Read the model definition and answer for the solid it produces. Units are mm, in the model's axes. Face numbers are marked on the shaded views. A direction names the side the tool comes from. Give positions to 0.01 mm unless a question says otherwise; leave off trailing zeros. Write each loop counter-clockwise with the first axis right and the second up, starting at its lowest first coordinate (ties: lowest second). Pieces come first, ordered by that corner, then holes.
```python
from build123d import *

# Parameters (mm, degrees)
SKETCH2_R           = 60.625
SKETCH2_R_2         = 45
BOSS_EXTRUDE1_DEPTH = 4.5
SKETCH3_R           = 49
SKETCH3_R_2         = 45
BOSS_EXTRUDE2_DEPTH = 52
SKETCH4_W           = 13.25
SKETCH4_H           = 8
SKETCH4_W_2         = 8
SKETCH4_H_2         = 38.5
BOSS_EXTRUDE3_DEPTH = 13
SKETCH5_W           = 10
SKETCH5_H           = 20
CUT_EXTRUDE1_DEPTH  = 26
SKETCH6_R           = 5
CUT_EXTRUDE2_DEPTH  = 50.375
SKETCH7_R           = 1.3
CUT_EXTRUDE3_DEPTH  = 7.2
BOSS_EXTRUDE4_DEPTH = 4
FILLET1_R           = 1
SKETCH9_R           = 2.5
CUT_EXTRUDE4_DEPTH  = 5.5000001


with BuildPart() as part:
    # Sketch2 → Boss-Extrude1 (new body)
    with BuildSketch(Plane(origin=(0, 0, 0), x_dir=(1, 0, 0), z_dir=(0, 1, 0))):
        Circle(SKETCH2_R)
        Circle(SKETCH2_R_2, mode=Mode.SUBTRACT)
    extrude(amount=BOSS_EXTRUDE1_DEPTH)

    # Sketch3 → Boss-Extrude2 (add)
    with BuildSketch(Plane(origin=(0, 4.5, 0), x_dir=(1, 0, 0), z_dir=(0, 1, 0))):
        Circle(SKETCH3_R)
        Circle(SKETCH3_R_2, mode=Mode.SUBTRACT)
    extrude(amount=BOSS_EXTRUDE2_DEPTH)

    # Sketch4 → Boss-Extrude3 (add, symmetric)
    with BuildSketch(Plane(origin=(0, 0, 0), x_dir=(0, 0, -1), z_dir=(1, 0, 0))):
        Polygon((-31.75, 30.5), (-45, 30.5), (-45, 17.25), align=None)
        with Locations((-38.375, 34.5)):
            Rectangle(SKETCH4_W, SKETCH4_H)
        with Locations((15.25, 19.25)):
            Rectangle(SKETCH4_W_2, SKETCH4_H_2)
    extrude(amount=BOSS_EXTRUDE3_DEPTH, both=True)

    # Sketch5 → Cut-Extrude1 (cut)
    with BuildSketch(Plane.XY):
        with Locations((0, 19.5)):
            Rectangle(SKETCH5_W, SKETCH5_H)
    extrude(amount=-CUT_EXTRUDE1_DEPTH, mode=Mode.SUBTRACT)

    # Sketch6 → Cut-Extrude2 (cut, through all)
    with BuildSketch(Plane.XY.offset(-11.25)):
        with Locations((0, 14)):
            Circle(SKETCH6_R)
    extrude(amount=-CUT_EXTRUDE2_DEPTH, mode=Mode.SUBTRACT)

    # Sketch7 → Cut-Extrude3 (cut)
    with BuildSketch(Plane(origin=(0, 38.5, 0), x_dir=(1, 0, 0), z_dir=(0, 1, 0))):
        with Locations((-5, 13.75)):
            Circle(SKETCH7_R)
        with Locations((5, 13.75)):
            Circle(SKETCH7_R)
        with Locations((-5, -34.25)):
            Circle(SKETCH7_R)
        with Locations((5, -34.25)):
            Circle(SKETCH7_R)
    extrude(amount=-CUT_EXTRUDE3_DEPTH, mode=Mode.SUBTRACT)

    # Sketch8 → Boss-Extrude4 (add)
    with BuildSketch(Plane.XZ):
        with BuildLine():
            Line((13, -11.25), (-13, -11.25))
            Line((-13, -11.25), (-37.248431585, -25.249838503))
            ThreePointArc((-37.248431585, -25.249838503), (0, -45), (37.248431585, -25.249838503))
            Line((37.248431585, -25.249838503), (13, -11.25))
        make_face()
        with BuildLine():
            Line((-19.516660498, -24.25), (-24.906460381, -27.361802413))
            ThreePointArc((-24.906460381, -27.361802413), (0, -37), (24.906460381, -27.361802413))
            Line((24.906460381, -27.361802413), (19.516660498, -24.25))
            Line((19.516660498, -24.25), (-19.516660498, -24.25))
        make_face(mode=Mode.SUBTRACT)
    extrude(amount=-BOSS_EXTRUDE4_DEPTH)

    # Fillet1
    fillet1_edges = [part.edges().sort_by_distance(p)[0] for p in [
        (-49, 4.5, 0),
    ]]
    fillet(fillet1_edges, radius=FILLET1_R)

    # Sketch9 → Cut-Extrude4 (cut, through all)
    with BuildSketch(Plane(origin=(0, 4.5, 0), x_dir=(1, 0, 0), z_dir=(0, 1, 0))):
        with Locations((35, 42)):
            Circle(SKETCH9_R)
        with Locations((35, -42)):
            Circle(SKETCH9_R)
        with Locations((-35, -42)):
            Circle(SKETCH9_R)
        with Locations((-35, 42)):
            Circle(SKETCH9_R)
    extrude(amount=-CUT_EXTRUDE4_DEPTH, mode=Mode.SUBTRACT)


solid = part.part
```
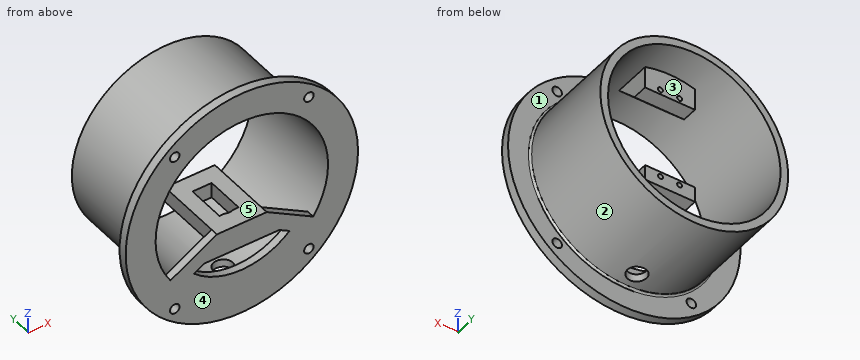
Item 1: Section D-D (y = 14) is taken. Write down the section's boundary in (x, z), and give its area (3 significant figures).
Result set:
outline: (-13, -19.25) - (-5, -19.25) - (-5, -11.25) - (-13, -11.25) - close; (-5, -48.74) - (-5, -44.72) arc R45 cw (long way) to (5, -44.72) - (5, -48.74) arc R49 ccw (long way) to start; (5, -19.25) - (13, -19.25) - (13, -11.25) - (5, -11.25) - close
area: 1,270 mm2
Item 2: Determine the mould class of the marked faces 1, 2 and 3 for opening direction X: pulls with the +X half, pulls with the -X half, needs draft (parallel to the pull), parting line crosses it, or undercut.
Result set:
face 1: needs draft
face 2: parting line crosses it
face 3: undercut
Item 3: Find the intervals of material crossed by line 1 along X through (y, z) = (30, 0); line 2 along Z through (x, y) = (-5, 33); line 3 along Z through (x, y) = (35, 1), in increasing order.
Result set:
line 1: x = -49 to -45, 45 to 49
line 2: z = -48.74 to -44.72, -19.25 to -15.05, -12.45 to -11.25, 31.75 to 32.95, 35.55 to 48.74
line 3: z = -49.5 to -44.5, -39.5 to -23.95, 28.28 to 39.5, 44.5 to 49.5
Item 4: Section B-B (y = 47) is taken. Write down the section's boundary in (x, z).
Result set:
outline: circle Ø98 at (0, 0); hole circle Ø90 at (0, 0)
Item 5: Which of the six approach directions +Z, -Z, +X, -X, +Y, -Y give full straight-line access (tool end or side, diameter ignored) to the marked faces 4 and 5?
Result set:
face 4: +Z, -Z, +X, -X, -Y
face 5: +Y, -Y
Item 6: Each of these flat-tipped pins is pushed along its axis until it touches: pin 1 Ø0.8 at (x, z) = (3.5, -16) entering from +Y; pin 2 Ø3.5 at (x, z) = (-5, -13.75) entering from -Y; pin 3 Ø8 at (x, y) = (6, 13) entering from +Z; pin 4 Ø8 at (x, y) = (-47.5, 25) entering from -Z. Where does it stop, or does it pass through?
Result set:
pin 1: stops at y = 38.5
pin 2: stops at y = 0
pin 3: stops at z = 48.96
pin 4: stops at z = -22.56
Item 7: Section A-A (y = 33) is taken. Write down the section's boundary in (x, z).
Result set:
outline: circle Ø98 at (0, 0); (-13, -19.25) - (13, -19.25) - (13, -11.25) - (-13, -11.25) - close; hole (-13, 31.75) - (-13, 43.08) arc R45 ccw (long way) to (13, 43.08) - (13, 31.75) - close; hole circle Ø2.6 at (-5, -13.75); hole circle Ø2.6 at (-5, 34.25); hole circle Ø2.6 at (5, -13.75); hole circle Ø2.6 at (5, 34.25)
Item 8: Section C-C (x = 35) is taken. Give the number of separate pieces and of enclosed holes in the cut face, and give its area (3 significant figures).
Result set:
separate pieces: 4
enclosed holes: 0
area: 789 mm2
